from build123d import *

# Parameters (mm, degrees)
BOSS_EXTRUDE1_DEPTH = 100
BOSS_EXTRUDE2_DEPTH = 50
DRAFT1_ANGLE        = 10


with BuildPart() as part:
    # Sketch1 → Boss-Extrude1 (new body)
    with BuildSketch(Plane.XY):
        with BuildLine():
            Line((0, 150), (0, -150))
            ThreePointArc((0, -150), (150, 0), (0, 150))
        make_face()
    extrude(amount=BOSS_EXTRUDE1_DEPTH)

    # Sketch2 → Boss-Extrude2 (add)
    with BuildSketch(Plane.ZY):
        Polygon((0, 180), (0, -180), (-81.642618236, -122.255018507), (-138.037816677, 121.301097394), align=None)
    extrude(amount=-BOSS_EXTRUDE2_DEPTH)

    # Draft1
    draft1_faces = [part.faces().sort_by_distance(p)[0] for p in [
        (25, -151.127509253, -40.821309118),
        (25, 150.650548697, -69.018908338),
        (25, -0.476960556, -109.840217456),
    ]]
    draft(draft1_faces, Plane(origin=(0, 0, 0), x_dir=(0, 0, 1), z_dir=(1, 0, 0)), DRAFT1_ANGLE)


solid = part.part
Build history of the part. All positions in model axes, mm. A direction names the side the tool comes from. Round coordinates to 2 decimals unless told otherwise and drop trailing zeros. Write each loop counter-clockwise with the first axis right and the second up, starting at its lowest first coordinate (ties: lowest second). Pieces come first, ordered by that corner, then holes. Notation, with made-up numbers: M 44,26.5 L 67,26.5 A17 cw 67,59.5 Z; hole C 58,28 d7. An arc over 180 degrees is marked long. Answer as a JSON object with one key per item and string values. Group by question number.
(1) Which spindle directions (+Z, -Z, +X, -X, +Y, -Y) get a long thin tool onto all of the face, cutting with end or side? Do faces 1 (the cylindrical face through (149.964, -3.298, 49.3)), 2 (the flat face through (88, 2, 0)), 3 (the flat face through (24.65, -147.983, -37.74)). Say none if no direction does.
(2) Cut at A-A (x = 12.5). Give the cut face in (y, z).
(3) Cut at C-C (z = -27.5). Give the cut face in (x, y), and give its area (3 significant figures).
(4) Cut at B-B (y = 77). Give the cut face in (x, z), and give its area (3 significant figures).
(5) Flat gauge pins, fed straight in: pin 1 (2 mm diameter, centred on x = 42, y = -41, fed in from -Z); pin 2 (1 mm diameter, centred on y = -107, z = -39.5, fed in from +X); pin 3 (19.5 mm diameter, centred on x = 33, y = -157.5, fed in from +Z). Where does each tip first touch, or does it go through?
(6) Drill centre lines: L1, parallel to Z at x = 67, y = -109; L2, parallel to X at y = -58.5, z = -10.5; L3, parallel to Z at x = 37, y = 121.5. Where is each one in solid material? Low to high.
(7) Cut at D-D (y = -104.5). Give the cut face in (x, z).
Responses:
{
 "1": {"face 1": "+Z, +X", "face 2": "-Z, +X, +Y, -Y", "face 3": "-Z, +X, -Y"},
 "2": {"outline": "M -177.3,0 L -120.94,-79.68 L 120,-135.47 L 177.6,0 L 149.48,0 L 149.48,100 L -149.48,100 L -149.48,0 Z"},
 "3": {"outline": "M 0,-160.55 L 50,-149.75 L 50,158.73 L 0,168.31 Z", "area": "15,900 mm2"},
 "4": {"outline": "M 0,-127.78 L 50,-118.73 L 50,0 L 128.73,0 L 128.73,100 L 0,100 Z", "area": "19,000 mm2"},
 "5": {"pin 1": "stops at z = -93.15", "pin 2": "stops at x = 50", "pin 3": "stops at z = 0"},
 "6": {"L1": "z = 0 to 100", "L2": "x = 0 to 50", "L3": "z = -120.9 to 100"},
 "7": {"outline": "M 0,-85.75 L 50,-76.7 L 50,0 L 107.61,0 L 107.61,100 L 0,100 Z"}
}
